```python
from build123d import *

# Parameters (mm, degrees)
F0_R         = 1.5
F1_DEPTH     = 4
F2_T1_DEPTH  = 15
F2_T3_DEPTH  = 70
F2_T5_DEPTH  = 7
F2_T7_DEPTH  = 10
F2_T9_DEPTH  = 16
F2_T11_DEPTH = 44
F2_T13_DEPTH = 16
F2_T15_DEPTH = 7
F2_T25_DEPTH = 12
F2_T29_DEPTH = 15
F2_T36_DEPTH = 15
F2_T40_DEPTH = 49
F2_T47_DEPTH = 49
F2_T51_DEPTH = 15
F2_T58_DEPTH = 15
F2_T62_DEPTH = 12


# Not quite as in the source:
# - a fillet or chamfer that OpenCascade refuses, or shapes differently, is made with other operations: its cross-section is extruded or revolved along the edge and cut away or added


with BuildPart() as f1:
    # F0 (on Front) → F1 (new body)
    with BuildSketch(Plane.XZ):
        Polygon((-55, 5), (-55, 0), (5, 0), (5, 5), (3, 5), (3, 10), (-3, 10), (-3, 5), (-47, 5), (-47, 10), (-53, 10), (-53, 5), align=None)
        with Locations((-50, 7.5)):
            Circle(F0_R, mode=Mode.SUBTRACT)
        with Locations((0, 7.5)):
            Circle(F0_R, mode=Mode.SUBTRACT)
    extrude(amount=F1_DEPTH)

    # F2: fillet of radius 2 on 14 edges, made by hand

    # F2_s2 → F2_t1 (cut)
    with BuildSketch(Plane.XY.offset(-5)):
        with BuildLine():
            ThreePointArc((-55, -2), (-54.4142135624, -3.4142135624), (-53, -4))
            Line((-53, -4), (-55, -4))
            Line((-55, -4), (-55, -2))
        make_face()
        with BuildLine():
            ThreePointArc((5, -2), (4.4142135624, -3.4142135624), (3, -4))
            Line((3, -4), (5, -4))
            Line((5, -4), (5, -2))
        make_face()
    extrude(amount=F2_T1_DEPTH, mode=Mode.SUBTRACT)

    # F2_s4 → F2_t3 (cut)
    with BuildSketch(Plane.YZ.offset(-60)):
        with BuildLine():
            ThreePointArc((-2, 0), (-3.4142135624, 0.5857864376), (-4, 2))
            Line((-4, 2), (-4, 0))
            Line((-4, 0), (-2, 0))
        make_face()
    extrude(amount=F2_T3_DEPTH, mode=Mode.SUBTRACT)

    # F2_s6 → F2_t5 (cut)
    with BuildSketch(Plane.YZ.offset(3)):
        with BuildLine():
            ThreePointArc((-2, 5), (-3.4142135624, 4.4142135624), (-4, 3))
            Line((-4, 3), (-4, 5))
            Line((-4, 5), (-2, 5))
        make_face()
    extrude(amount=F2_T5_DEPTH, mode=Mode.SUBTRACT)

    # F2_s8 → F2_t7 (cut)
    with BuildSketch(Plane.XY.offset(5)):
        with BuildLine():
            ThreePointArc((3, -2), (2.4142135624, -3.4142135624), (1, -4))
            Line((1, -4), (3, -4))
            Line((3, -4), (3, -2))
        make_face()
        with BuildLine():
            ThreePointArc((-3, -2), (-2.4142135624, -3.4142135624), (-1, -4))
            Line((-1, -4), (-3, -4))
            Line((-3, -4), (-3, -2))
        make_face()
        with BuildLine():
            ThreePointArc((-47, -2), (-47.5857864376, -3.4142135624), (-49, -4))
            Line((-49, -4), (-47, -4))
            Line((-47, -4), (-47, -2))
        make_face()
        with BuildLine():
            ThreePointArc((-53, -2), (-52.4142135624, -3.4142135624), (-51, -4))
            Line((-51, -4), (-53, -4))
            Line((-53, -4), (-53, -2))
        make_face()
    extrude(amount=F2_T7_DEPTH, mode=Mode.SUBTRACT)

    # F2_s10 → F2_t9 (cut)
    with BuildSketch(Plane.YZ.offset(-8)):
        with BuildLine():
            ThreePointArc((-2, 10), (-3.4142135624, 9.4142135624), (-4, 8))
            Line((-4, 8), (-4, 10))
            Line((-4, 10), (-2, 10))
        make_face()
    extrude(amount=F2_T9_DEPTH, mode=Mode.SUBTRACT)

    # F2_s12 → F2_t11 (cut)
    with BuildSketch(Plane.YZ.offset(-47)):
        with BuildLine():
            ThreePointArc((-2, 5), (-3.4142135624, 4.4142135624), (-4, 3))
            Line((-4, 3), (-4, 5))
            Line((-4, 5), (-2, 5))
        make_face()
    extrude(amount=F2_T11_DEPTH, mode=Mode.SUBTRACT)

    # F2_s14 → F2_t13 (cut)
    with BuildSketch(Plane.YZ.offset(-58)):
        with BuildLine():
            ThreePointArc((-2, 10), (-3.4142135624, 9.4142135624), (-4, 8))
            Line((-4, 8), (-4, 10))
            Line((-4, 10), (-2, 10))
        make_face()
    extrude(amount=F2_T13_DEPTH, mode=Mode.SUBTRACT)

    # F2_s16 → F2_t15 (cut)
    with BuildSketch(Plane.YZ.offset(-60)):
        with BuildLine():
            ThreePointArc((-2, 5), (-3.4142135624, 4.4142135624), (-4, 3))
            Line((-4, 3), (-4, 5))
            Line((-4, 5), (-2, 5))
        make_face()
    extrude(amount=F2_T15_DEPTH, mode=Mode.SUBTRACT)

    # F2_s17 → F2_t18 (revolve, cut)
    with BuildSketch(Plane.XY.offset(7.5)):
        with BuildLine():
            ThreePointArc((-48.5, -2), (-47.9142135624, -3.4142135624), (-46.5, -4))
            Line((-46.5, -4), (-48.5, -4))
            Line((-48.5, -4), (-48.5, -2))
        make_face()
    revolve(axis=Axis((-50, -4, 7.5), (0, -1, 0)), mode=Mode.SUBTRACT)

    # F2_s19 → F2_t20 (revolve, cut)
    with BuildSketch(Plane.XY.offset(7.5)):
        with BuildLine():
            ThreePointArc((1.5, -2), (2.0857864376, -3.4142135624), (3.5, -4))
            Line((3.5, -4), (1.5, -4))
            Line((1.5, -4), (1.5, -2))
        make_face()
    revolve(axis=Axis((0, -4, 7.5), (0, -1, 0)), mode=Mode.SUBTRACT)


with BuildPart() as f2_tool23:
    # F2_s24 → F2_t25 (new body)
    with BuildSketch(Plane.YZ.offset(10)):
        with BuildLine():
            ThreePointArc((-2, 5), (-3.4142135624, 4.4142135624), (-4, 3))
            Line((-4, 3), (-4, 5))
            Line((-4, 5), (-2, 5))
        make_face()
    extrude(amount=-F2_T25_DEPTH)

    split(bisect_by=Plane.YZ.offset(3), keep=Keep.BOTTOM)


with BuildPart() as f2_tool27:
    # F2_s28 → F2_t29 (new body)
    with BuildSketch(Plane.XY):
        with BuildLine():
            ThreePointArc((3, -2), (2.4142135624, -3.4142135624), (1, -4))
            Line((1, -4), (3, -4))
            Line((3, -4), (3, -2))
        make_face()
    extrude(amount=F2_T29_DEPTH)

    split(bisect_by=Plane.XY.offset(5), keep=Keep.BOTTOM)


with BuildPart() as f2_tool23_1:
    add(f2_tool23.part)

    # F2_t31: intersect F2_tool27
    add(f2_tool27.part, mode=Mode.INTERSECT)


with BuildPart() as f1_1:
    add(f1.part)

    # F2_t21: cut F2_tool23
    add(f2_tool23_1.part, mode=Mode.SUBTRACT)


with BuildPart() as f2_tool34:
    # F2_s35 → F2_t36 (new body)
    with BuildSketch(Plane.XY.offset(15)):
        with BuildLine():
            ThreePointArc((-3, -2), (-2.4142135624, -3.4142135624), (-1, -4))
            Line((-1, -4), (-3, -4))
            Line((-3, -4), (-3, -2))
        make_face()
    extrude(amount=-F2_T36_DEPTH)

    split(bisect_by=Plane.XY.offset(5), keep=Keep.BOTTOM)


with BuildPart() as f2_tool38:
    # F2_s39 → F2_t40 (new body)
    with BuildSketch(Plane.YZ.offset(2)):
        with BuildLine():
            ThreePointArc((-2, 5), (-3.4142135624, 4.4142135624), (-4, 3))
            Line((-4, 3), (-4, 5))
            Line((-4, 5), (-2, 5))
        make_face()
    extrude(amount=-F2_T40_DEPTH)

    split(bisect_by=Plane.YZ.offset(-3), keep=Keep.TOP)


with BuildPart() as f2_tool34_1:
    add(f2_tool34.part)

    # F2_t42: intersect F2_tool38
    add(f2_tool38.part, mode=Mode.INTERSECT)


with BuildPart() as f1_2:
    add(f1_1.part)

    # F2_t32: cut F2_tool34
    add(f2_tool34_1.part, mode=Mode.SUBTRACT)


with BuildPart() as f2_tool45:
    # F2_s46 → F2_t47 (new body)
    with BuildSketch(Plane.YZ.offset(-3)):
        with BuildLine():
            ThreePointArc((-2, 5), (-3.4142135624, 4.4142135624), (-4, 3))
            Line((-4, 3), (-4, 5))
            Line((-4, 5), (-2, 5))
        make_face()
    extrude(amount=-F2_T47_DEPTH)

    split(bisect_by=Plane.YZ.offset(-47), keep=Keep.BOTTOM)


with BuildPart() as f2_tool49:
    # F2_s50 → F2_t51 (new body)
    with BuildSketch(Plane.XY):
        with BuildLine():
            ThreePointArc((-47, -2), (-47.5857864376, -3.4142135624), (-49, -4))
            Line((-49, -4), (-47, -4))
            Line((-47, -4), (-47, -2))
        make_face()
    extrude(amount=F2_T51_DEPTH)

    split(bisect_by=Plane.XY.offset(5), keep=Keep.BOTTOM)


with BuildPart() as f2_tool45_1:
    add(f2_tool45.part)

    # F2_t53: intersect F2_tool49
    add(f2_tool49.part, mode=Mode.INTERSECT)


with BuildPart() as f1_3:
    add(f1_2.part)

    # F2_t43: cut F2_tool45
    add(f2_tool45_1.part, mode=Mode.SUBTRACT)


with BuildPart() as f2_tool56:
    # F2_s57 → F2_t58 (new body)
    with BuildSketch(Plane.XY.offset(15)):
        with BuildLine():
            ThreePointArc((-53, -2), (-52.4142135624, -3.4142135624), (-51, -4))
            Line((-51, -4), (-53, -4))
            Line((-53, -4), (-53, -2))
        make_face()
    extrude(amount=-F2_T58_DEPTH)

    split(bisect_by=Plane.XY.offset(5), keep=Keep.BOTTOM)


with BuildPart() as f2_tool60:
    # F2_s61 → F2_t62 (new body)
    with BuildSketch(Plane.YZ.offset(-48)):
        with BuildLine():
            ThreePointArc((-2, 5), (-3.4142135624, 4.4142135624), (-4, 3))
            Line((-4, 3), (-4, 5))
            Line((-4, 5), (-2, 5))
        make_face()
    extrude(amount=-F2_T62_DEPTH)

    split(bisect_by=Plane.YZ.offset(-53), keep=Keep.TOP)


with BuildPart() as f2_tool56_1:
    add(f2_tool56.part)

    # F2_t64: intersect F2_tool60
    add(f2_tool60.part, mode=Mode.INTERSECT)


with BuildPart() as f1_4:
    add(f1_3.part)

    # F2_t54: cut F2_tool56
    add(f2_tool56_1.part, mode=Mode.SUBTRACT)


solid = f1_4.part
```
Check sheet for the modelled part. Datum: model origin and axes. Units: mm. A direction names the side the tool comes from. Give positions to 0.01 mm unless a question says otherwise; leave off trailing zeros. Loops run counter-clockwise (first coordinate to the right, second up) from the corner with the lowest first, then second, coordinate; pieces in that order, holes last. Notation, with made-up numbers: M -11.5,9 L 16.5,9 A18 ccw 16.5,33 Z; hole C 2,73.5 d10. An arc over 180 degrees is marked long. Answer as CSV lines item,"result".
Item 1: Scan lines: L1, parallel to Z at x = -50, y = -0.45; L2, parallel to X at y = -1.6, z = 8.5; L3, parallel to X at y = -2.45, z = 8.75. Record each from-to range of solid material in increasing order.
Reply:
L1,"0 to 6, 9 to 10"
L2,"-53 to -51.12, -48.88 to -47, -3 to -1.12, 1.12 to 3"
L3,"-52.95 to -50.92, -49.08 to -47.05, -2.95 to -0.92, 0.92 to 2.95"
Item 2: Sectioned sample at C-C, the plane z = 7.5. Enter the section's corners in (x, y), then the cut area to 3 significant figures.
Reply:
outline,"M -53,-2 A2 ccw -52.25,-3.56 A2 ccw -51.5,-2 L -51.5,0 L -53,0 Z; M -48.5,-2 A2 ccw -47.75,-3.56 A2 ccw -47,-2 L -47,0 L -48.5,0 Z; M -3,-2 A2 ccw -2.25,-3.56 A2 ccw -1.5,-2 L -1.5,0 L -3,0 Z; M 1.5,-2 A2 ccw 2.25,-3.56 A2 ccw 3,-2 L 3,0 L 1.5,0 Z"
area,"18.5 mm^2"
Item 3: Sectioned sample at A-A, the plane y = -1.1. Enter the section's corners in (x, z).
Reply:
outline,"M -55,0 L 5,0 L 5,5 L 3,5 L 3,10 L -3,10 L -3,5 L -47,5 L -47,10 L -53,10 L -53,5 L -55,5 Z; hole C -50,7.5 d3; hole C 0,7.5 d3"
Item 4: Set-up check for faces 4 (the face through (-25, -1, 5)), 5 (the face through (-53, -1, 8)), 6 (the face through (-25.34, -3.4, 4.43)), 7 (the face through (2.65, -3.13, 6.45)), 8 (the face through (-52.65, -3.13, 6.45)): record each of +Z, -Z, +X, -X, +Y, -Y from which the full face is reachable in a straight line by a thin tool's end or side.
Reply:
face 4,"+Z, +Y, -Y"
face 5,"+Z, -X, +Y, -Y"
face 6,"+Z, -Y"
face 7,"+Z, +X, -Y"
face 8,"+Z, -X, -Y"
Item 5: Sectioned sample at B-B, the plane x = 0. Enter the section's corners in (y, z), then the cut area to 3 significant figures.
Reply:
outline,"M -4,2 A2 ccw -2,0 L 0,0 L 0,6 L -2,6 A2 ccw -4,4 Z; M -3.32,9.5 A2 ccw -2,9 L 0,9 L 0,10 L -2,10 A2 ccw Z"
area,"25.2 mm^2"
Item 6: Draft check along Z on faces 1 (the face through (-51.2, -1, 6.6)), 2 (the face through (4.65, -3.13, 2.46)), 3 (the face through (4, -1, 5)). Enter one of: pulls with the +Z half, pulls with the -Z half, needs draft (parallel to the pull), parting line crosses it, or undercut.
Reply:
face 1,"undercut"
face 2,"needs draft"
face 3,"pulls with the +Z half"
Item 7: Depth check by flat-ended pin: pin 1 Ø1.6 at (y, z) = (-1, 8.5) entering from -X; pin 2 Ø2 at (y, z) = (-1.5, 7) entering from +X; pin 3 Ø1.8 at (x, z) = (0, 7.5) entering from -Y; pin 4 Ø2 at (x, z) = (-41, 3.5) entering from -Y. Enter the tip coordinate at first touch or a pass-through.
Reply:
pin 1,"x = -53"
pin 2,"x = 3"
pin 3,"through"
pin 4,"y = -4"
Item 8: Sectioned sample at D-D, the plane x = -40. Enter the section's corners in (y, z).
Reply:
outline,"M -4,2 A2 ccw -2,0 L 0,0 L 0,5 L -2,5 A2 ccw -4,3 Z"
